Design review of the part built by this model. Coordinates are the model's own, in mm. Face numbers are marked on the shaded views. Round coordinates to 2 decimals unless told otherwise and drop trailing zeros. Write each loop counter-clockwise with the first axis right and the second up, starting at its lowest first coordinate (ties: lowest second). Pieces come first, ordered by that corner, then holes. Notation, with made-up numbers: (87.5, -7.75) -> (144.5, -7.75) arc R27 ccw to (144.5, 25.25) -> close; hole circle Ø5 at (-31, -36). An arc over 180 degrees is marked (long way). Write item = value, one per line. Start each with the question number.
Item 1: Add section C-C, the plane y = 2.05. State the section outline as (x, z) points.
Item 2: To check wall thickness, follow L1, parallel to X at y = 3.2, z = 0; L2, parallel to X at y = 3.7, z = 0; L3, parallel to Z at x = -1, y = 3.8. State the ranges of each line that lie inside material, in increasing order.
Item 3: For pin 1 Ø2 at (x, y) = (-4.5, 3) entering from +Z; pin 2 Ø2 at (y, z) = (2.5, -3.5) entering from -X; pin 3 Ø2 at (x, y) = (5.5, 3) entering from +Z; pin 4 Ø7 at (x, z) = (-2, 0.5) entering from -Y, all flat-tipped, find the tip position at first contact; note any pin that passes through.
Item 4: Mouldability with a two-part tool opening along X and no side actions: class the marked faces 1 and 2 as released by +X, released by -X, zero draft, split by the parting line, or undercut.
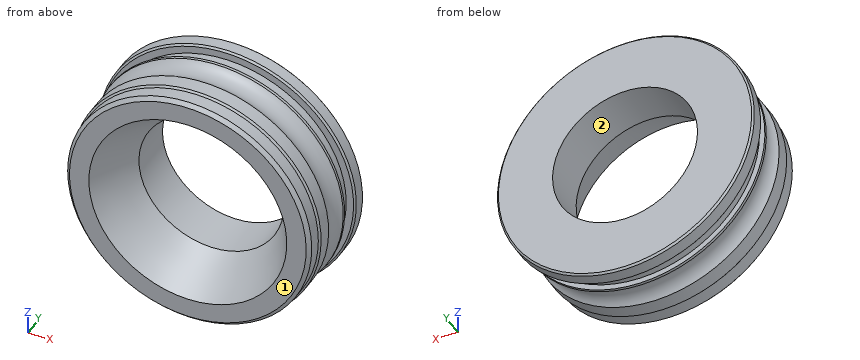
from build123d import *


with BuildPart() as part:
    # Croquis1 → Revolución1 (revolve)
    with BuildSketch(Plane.XY, mode=Mode.PRIVATE) as revoluci_n1_sk:
        with BuildLine():
            Line((6.45, 0), (6.65, 0.2))
            Line((6.65, 0.2), (6.65, 0.9))
            Line((6.65, 0.9), (6.75, 1))
            Line((6.75, 1), (6.75, 1.667))
            Line((6.75, 1.667), (6.75, 1.8))
            ThreePointArc((6.75, 1.8), (6.46467894, 2.534577468), (6.8, 3.247719775))
            Line((6.8, 3.247719775), (6.8, 3.4))
            Line((6.8, 3.4), (6.5, 3.4))
            Line((6.5, 3.4), (6.5, 4.15))
            Line((6.5, 4.15), (6.9, 4.15))
            Line((6.9, 4.15), (7, 4.25))
            Line((7, 4.25), (7, 4.9))
            Line((7, 4.9), (6.9, 5))
            Line((6.9, 5), (3.95, 5))
            Line((3.95, 5), (3.95, 2.5))
            Line((3.95, 2.5), (5.393375673, 0))
            Line((5.393375673, 0), (6.45, 0))
        make_face()
    revolve(revoluci_n1_sk.sketch.rotate(Axis((0, 0, 0), (0, 1, 0)), 90), axis=Axis((0, 0, 0), (0, 1, 0)))


solid = part.part
Result set:
q1.outline = circle Ø13.14 at (0, 0); hole circle Ø8.42 at (0, 0)
q2.L1 = -6.75 to -3.95, 3.95 to 6.75
q2.L2 = -6.5 to -3.95, 3.95 to 6.5
q2.L3 = -6.42 to -3.82, 3.82 to 6.42
q3.pin_1 = 5.81
q3.pin_2 = -6.18
q3.pin_3 = 5.07
q3.pin_4 = 0
q4.face_1 = zero draft
q4.face_2 = undercut
